Print and shaded views of the part. All mm, measured from the part's lowest x, y and z. Give positions to 0.01 mm unless a question says otherwise; leave off trailing zeros. Write each loop counter-clockwise with the first axis right and the second up, starting at its lowest first coordinate (ties: lowest second). Pieces come first, ordered by that corner, then holes. Notation, with made-up numbers: (-25, -6) -> (11, -6) arc R18 ccw to (11, 5) -> close; hole circle Ø1 at (-9, -22.5). An arc over 180 degrees is marked (long way). Put each result on its own line as item: value.
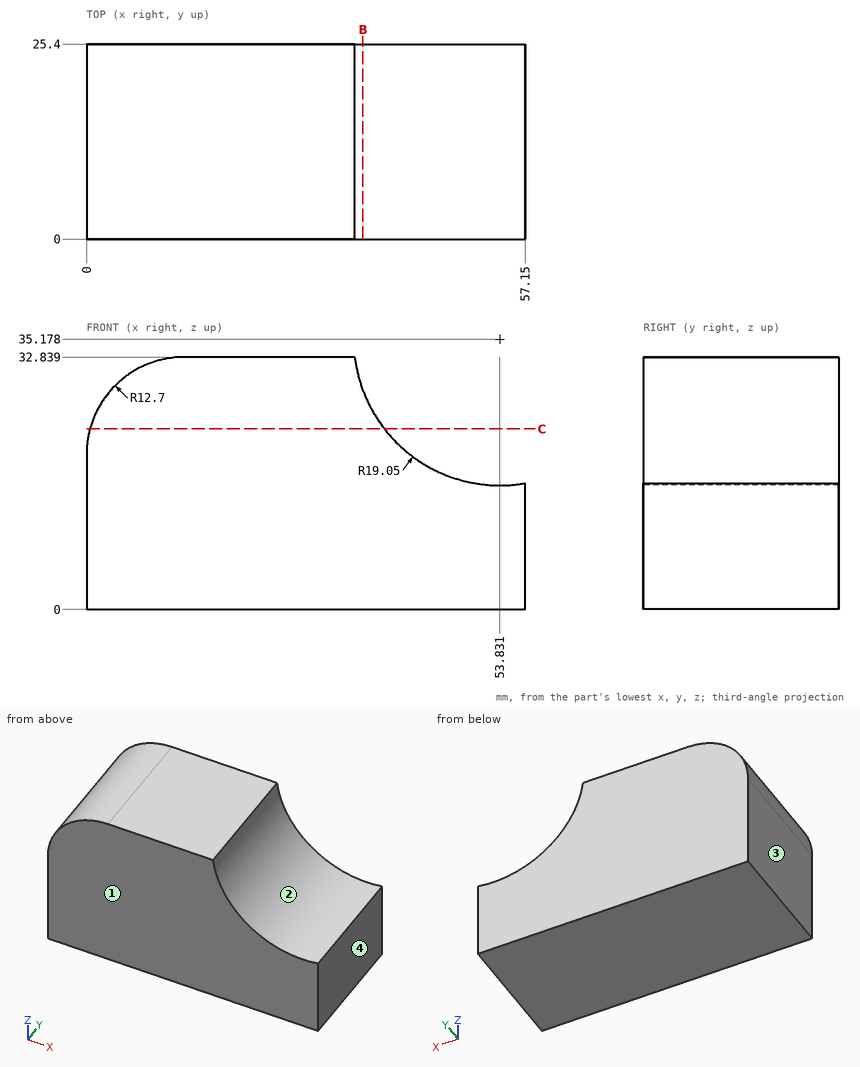
1) Pull direction X, two halves, no side cores. Call the marked faces 1, 2, 3 and 4: released by +X, released by -X, zero draft, split by the parting line, or undercut.
Filled sheet:
face 1: zero draft
face 2: undercut
face 3: released by -X
face 4: released by +X
2) Wall check: L1, parallel to Z at x = 54, y = 9; L2, parallel to X at y = 3.75, z = 21 (1 decimal); L3, parallel to X at y = 3.25, z = 31.5 (1 decimal). Give the ranges that are in metal, low to high.
Filled sheet:
L1: 0 to 16.13
L2: 0 to 41.1
L3: 7 to 35.1
3) Slice it at B-B (x = 36). Write the cut outline in (y, z).
Filled sheet:
outline: (0, 0) -> (25.4, 0) -> (25.4, 28.47) -> (0, 28.47) -> close
4) Slice it at C-C (z = 23.5). Write the cut outline in (x, y).
Filled sheet:
outline: (0.45, 0) -> (38.78, 0) -> (38.78, 25.4) -> (0.45, 25.4) -> close
5) Pin check, flat tip, straight feed: pin 1 (3 mm diameter, centred on y = 2.5, z = 28.5, fed in from +X) (1 decimal). Stop position of the tip, or through.
Filled sheet:
pin 1: x = 36.6
